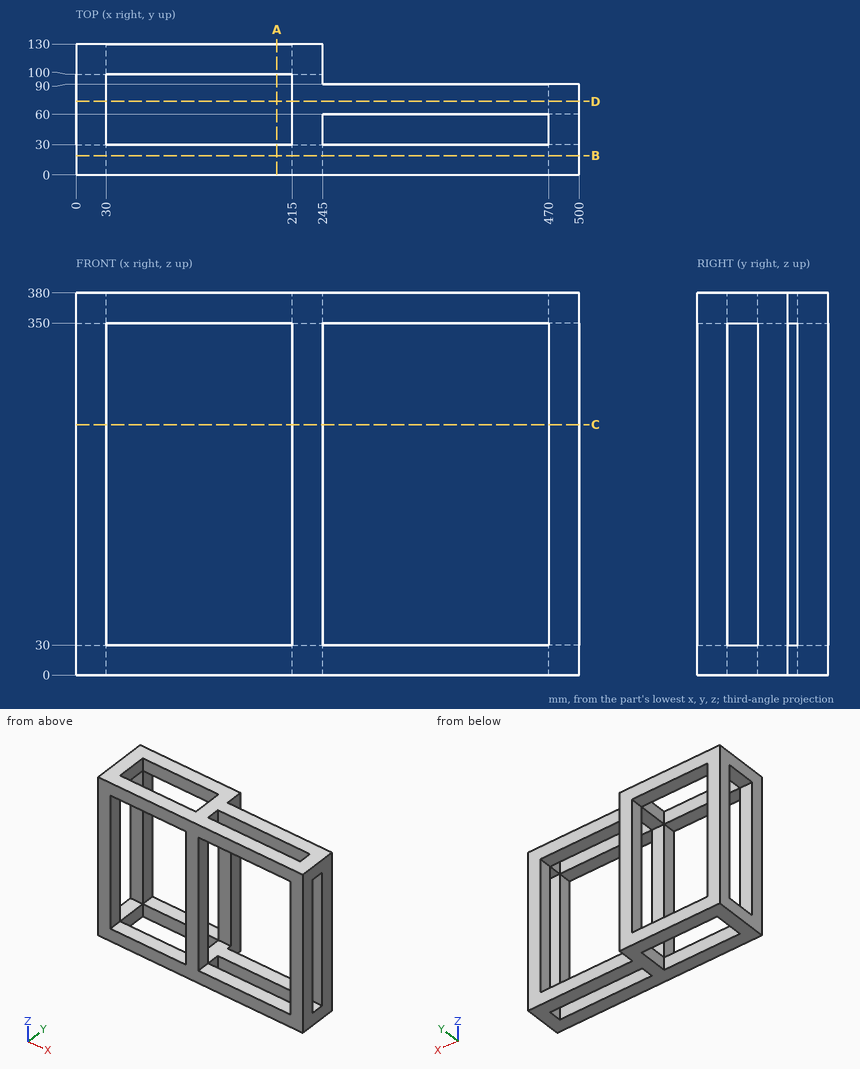
Study the drawing (mm; zero at the part's minimum x, y, z) and answer. Round coordinates to 2 decimals unless told otherwise and drop trailing zeros. Loops run counter-clockwise (first coordinate to the right, second up) from the corner with the lowest first, then second, coordinate; pieces in that order, holes last. Notation, with made-up numbers: (21, 37) -> (53, 37) arc R23 cw to (53, 50) -> close; hole circle Ø7 at (44, -17). An arc over 180 degrees is marked (long way). Write each question's results on one line, items separated by ' | '. Start each with the question number.
1. Section B-B (y = 19) is taken. Determine the outline of the cut face in (x, z).
2. Section C-C (z = 249) is taken. Determine the outline of the cut face in (x, y).
3. Section D-D (y = 73) is taken. Determine the outline of the cut face in (x, z).
4. Section A-A (x = 199.5) is taken. Determine the outline of the cut face in (y, z), plus the area to 3 significant figures.
5. Given pin 1 Ø9 at (x, z) = (357, 372.5) entering from -Y, flat-ended and moving along its own axis, determine where the tip first touches the part or whether it passes through.
6. Find the intervals of material crossed by probe 1 along X at (y, z) = (54.5, 15.5); probe 2 along Y at (x, z) = (50, 22); probe 3 along Z at (x, y) = (104, 20), in increasing order. Write a range as from..to.
Evaluation:
1) outline: (0, 0) -> (500, 0) -> (500, 380) -> (0, 380) -> close; hole (30, 30) -> (215, 30) -> (215, 350) -> (30, 350) -> close; hole (245, 30) -> (470, 30) -> (470, 350) -> (245, 350) -> close
2) outline: (0, 0) -> (30, 0) -> (30, 30) -> (0, 30) -> close; (0, 100) -> (30, 100) -> (30, 130) -> (0, 130) -> close; (215, 0) -> (245, 0) -> (245, 30) -> (215, 30) -> close; (215, 100) -> (245, 100) -> (245, 130) -> (215, 130) -> close; (470, 0) -> (500, 0) -> (500, 30) -> (470, 30) -> close; (470, 60) -> (500, 60) -> (500, 90) -> (470, 90) -> close
3) outline: (0, 0) -> (30, 0) -> (30, 30) -> (0, 30) -> close; (0, 350) -> (30, 350) -> (30, 380) -> (0, 380) -> close; (215, 0) -> (500, 0) -> (500, 380) -> (215, 380) -> (215, 350) -> (470, 350) -> (470, 30) -> (215, 30) -> close
4) outline: (0, 0) -> (30, 0) -> (30, 30) -> (0, 30) -> close; (0, 350) -> (30, 350) -> (30, 380) -> (0, 380) -> close; (100, 0) -> (130, 0) -> (130, 30) -> (100, 30) -> close; (100, 350) -> (130, 350) -> (130, 380) -> (100, 380) -> close | area: 3,600 mm2
5) pin 1: stops at y = 0
6) probe 1: x = 0..30, 215..245, 470..500 | probe 2: y = 0..30, 100..130 | probe 3: z = 0..30, 350..380
